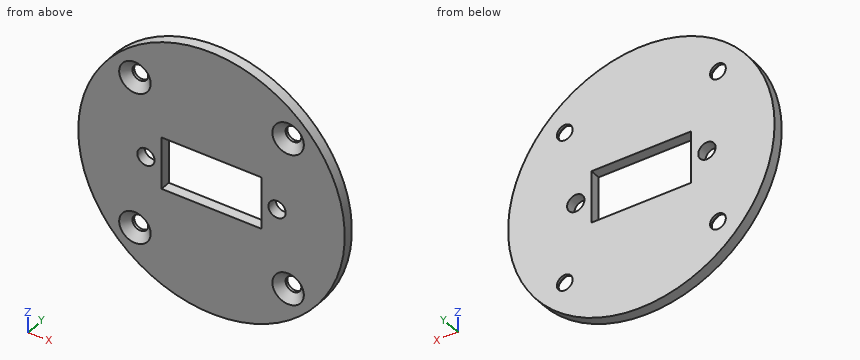
Autodesk Inventor part; units mm, degrees
ref_plane "YZ Plane" through (0, 0, 0) normal (1, 0, 0) x (0, 1, 0)
ref_plane "XZ Plane" through (0, 0, 0) normal (0, 1, 0) x (-1, 0, 0)
ref_plane "XY Plane" through (0, 0, 0) normal (0, 0, 1) x (1, 0, 0)
sketch "Skizze1" plane through (0, 0, 0) normal (0, 1, 0) x (-1, 0, 0)
  circle A0 centre (0, 0) radius 25.4
  dimension "d0" = 50.8
extrude "Extrusion1" add sketch "Skizze1" along normal blind 2
sketch "Skizze2" plane through (0, 0, 0) normal (0, -1, 0) x (1, 0, 0)
  circle A0 centre (0, 0) radius 25.4
  line L0 (-14.6, 14.6) -> (14.6, 14.6) construction
  line L1 (14.6, 14.6) -> (14.6, -14.6) construction
  line L2 (14.6, -14.6) -> (-14.6, -14.6) construction
  line L3 (-14.6, -14.6) -> (-14.6, 14.6) construction
  line L4 (0, 0) -> (14.6, 0) construction
  line L5 (0, 0) -> (0, 14.6) construction
  dimension "d3" = 29.2
  dimension "d4" = 29.2
hole "Bohrung1" at (-14.6, 0, 14.6) at (14.6, 0, 14.6) at (14.6, 0, -14.6) at (-14.6, 0, -14.6) direction (0, 1, 0) diameter 3 end through all countersink diameter 6 countersink angle 90
sketch "Skizze7" plane through (0, 0, 0) normal (0, -1, 0) x (1, 0, 0)
  circle A0 centre (0, 0) radius 25.4
  line L0 (-9.5, 5) -> (9.5, 5)
  line L1 (9.5, 5) -> (9.5, -5)
  line L2 (9.5, -5) -> (-9.5, -5)
  line L3 (-9.5, -5) -> (-9.5, 5)
  line L4 (0, 0) -> (9.5, 0) construction
  line L5 (0, 0) -> (0, 5) construction
  line L6 (0, 0) -> (12.5, 0) construction
  line L7 (0, 0) -> (-12.5, 0) construction
  dimension "d25" = 19
  dimension "d26" = 10
  dimension "d28" = 12.5
  dimension "d29" = 12.5
extrude "Extrusion5" cut sketch "Skizze7" against normal blind 2 contours L0 L1 L2 L3
sketch "Skizze8" plane through (0, 0, 0) normal (0, -1, 0) x (1, 0, 0)
  circle A0 centre (0, 0) radius 25.4
  line L0 (0, 0) -> (12.5, 0) construction
  line L1 (0, 0) -> (-12.5, 0) construction
  dimension "d32" = 12.5
  dimension "d33" = 12.5
hole "Bohrung2" at (-12.5, 0, 0) at (12.5, 0, 0) direction (0, 1, 0) diameter 3.3 end through all
properties part number "anschluss_daten_1"
Part model, mm, in its own coordinate system. Coordinates: 2 decimals unless noted, no trailing zeros. Loops run counter-clockwise (first coordinate to the right, second up) from the corner with the lowest first, then second, coordinate; pieces in that order, holes last. Notation, with made-up numbers: (87, -40) - (94, -40) arc R15 cw to (94, -28) - close; hole circle Ø8 at (22.5, 68). An arc over 180 degrees is marked (long way). Write item = value, one per line. Start each with the question number.
Item 1: Wall check: L1, parallel to X at y = 0.6, z = -14; L2, parallel to Z at x = 15, y = 1.8; L3, parallel to Z at x = -14.6, y = 1.85. Give the ranges that are in metal, low to high. Write a range as from..to.
Item 2: Cut at B-B, the plane z = 0. Give the cut face in (x, y).
Item 3: Flat gauge pins, fed straight in: pin 1 Ø1 at (x, y) = (-3.5, 1.5) entering from +Z; pin 2 Ø0.6 at (y, z) = (1, -2.5) entering from +X; pin 3 Ø1 at (y, z) = (1.5, 18) entering from +X. Where does each tip first touch, or does it go through?
Item 4: Cut at A-A, the plane y = 0.4. Give the cut face in (x, z), and give its area (3 significant figures).
Item 5: Cut at D-D, the plane z = -14.6. Give the cut face in (x, y).
Item 6: Cut at C-C, the plane x = 3. Give the cut face in (y, z).
The answers:
q1.L1 = -21.19..-16.92, -12.28..12.28, 16.92..21.19
q1.L2 = -20.5..-16.05, -13.15..13.15, 16.05..20.5
q1.L3 = -20.78..-16.1, -13.1..13.1, 16.1..20.78
q2.outline = (-25.4, 0) - (-14.15, 0) - (-14.15, 2) - (-25.4, 2) - close; (-10.85, 0) - (-9.5, 0) - (-9.5, 2) - (-10.85, 2) - close; (9.5, 0) - (10.85, 0) - (10.85, 2) - (9.5, 2) - close; (14.15, 0) - (25.4, 0) - (25.4, 2) - (14.15, 2) - close
q3.pin_1 = 25.22
q3.pin_2 = 25.3
q3.pin_3 = 18.41
q4.outline = circle Ø50.8 at (0, 0); hole circle Ø5.2 at (-14.6, -14.6); hole circle Ø5.2 at (-14.6, 14.6); hole circle Ø3.3 at (-12.5, 0); hole (-9.5, -5) - (9.5, -5) - (9.5, 5) - (-9.5, 5) - close; hole circle Ø3.3 at (12.5, 0); hole circle Ø5.2 at (14.6, -14.6); hole circle Ø5.2 at (14.6, 14.6)
q4.area = 1,730 mm2
q5.outline = (-20.78, 0) - (-17.6, 0) - (-16.1, 1.5) - (-16.1, 2) - (-20.78, 2) - close; (-13.1, 1.5) - (-11.6, 0) - (11.6, 0) - (13.1, 1.5) - (13.1, 2) - (-13.1, 2) - close; (16.1, 1.5) - (17.6, 0) - (20.78, 0) - (20.78, 2) - (16.1, 2) - close
q6.outline = (0, -25.22) - (2, -25.22) - (2, -5) - (0, -5) - close; (0, 5) - (2, 5) - (2, 25.22) - (0, 25.22) - close
